Autodesk Inventor part; units mm, degrees
ref_plane "YZ Plane" through (0, 0, 0) normal (1, 0, 0) x (0, 1, 0)
ref_plane "XZ Plane" through (0, 0, 0) normal (0, 1, 0) x (-1, 0, 0)
ref_plane "XY Plane" through (0, 0, 0) normal (0, 0, 1) x (1, 0, 0)
sketch "Sketch1" plane through (0, 0, 0) normal (0, 0, 1) x (1, 0, 0)
  line L0 (0, 4.0415) -> (3.5, 2.0207)
  line L1 (3.5, 2.0207) -> (3.5, -2.0207)
  line L2 (3.5, -2.0207) -> (0, -4.0415)
  line L3 (0, -4.0415) -> (-3.5, -2.0207)
  line L4 (-3.5, -2.0207) -> (-3.5, 2.0207)
  line L5 (-3.5, 2.0207) -> (0, 4.0415)
  point P0 (0, 0)
  point P1 (0, 0)
  dimension "d0" = 7
extrude "Extrusion1" add sketch "Sketch1" along normal blind 2.9
sketch "Sketch2" plane through (0, 0, 2.9) normal (0, 0, 1) x (1, 0, 0)
  circle A0 centre (0, 0) radius 2
  dimension "d3" = 4
extrude "Extrusion2" cut sketch "Sketch2" against normal blind 5
sketch "Sketch3" plane through (0, 0, 2.9) normal (0, 0, 1) x (1, 0, 0)
  circle A0 centre (0, 0) radius 3.5
  circle A1 centre (0, 0) radius 2
extrude "Extrusion3" add sketch "Sketch3" along normal blind 2.1
chamfer "Chamfer1" distance 0.2 angle 45 1 edges at (-2, 0, 0)
thread "Thread1"
chamfer "Chamfer2" distance 0.3 angle 45 1 edges at (-2, 0, 5)
properties part number "P88044_Nylor_Nut_M4"
The listing builds one solid part. Answer for the finished solid, in the listing's coordinates (mm). A direction names the side the tool comes from. Coordinates: 2 decimals unless noted, no trailing zeros. Write each loop counter-clockwise with the first axis right and the second up, starting at its lowest first coordinate (ties: lowest second). Pieces come first, ordered by that corner, then holes. Notation, with made-up numbers: (-2, 59) - (19, 59) arc R28 ccw to (19, 98) - close; hole circle Ø7 at (25, 25). An arc over 180 degrees is marked (long way). Return JSON: item names as keys, results as strings. Group by question number.
1. A cutting plane is placed at A-A, the plane z = 1.45. Determine the outline of the cut face in (x, y), plus the area to 3 significant figures.
2. Which of the six approach directions +Z, -Z, +X, -X, +Y, -Y give full straight-line access (tool end or side, diameter ignored) to faces 1 (the flat face through (-3.15, -1.85, 2.9)), 2 (the flat face through (3.2, -1.8, 2.9)), 3 (the cylindrical face through (3.233, 1.341, 3.935))?
3. A cutting plane is placed at D-D, the plane z = 3.1. Determine the outline of the cut face in (x, y), plus the area to 3 significant figures.
4. A cutting plane is placed at B-B, the plane y = 3.25. Determine the outline of the cut face in (x, z).
5. Straight lines are drawn through the part: L1, parallel to Y at x = 0, z = 3.45; L2, parallel to X at y = -0.5, z = 1.7; L3, parallel to Y at x = -0.75, z = 2.3. For each, find the intervals that lie inside material, in ascending order.
6. Given pin 1 (1.5 mm diameter, centred on x = 1, y = 0.5, fed in from +Z); pin 2 (1.1 mm diameter, centred on x = 0.5, y = 3.5, fed in from +Z); pin 3 (1 mm diameter, centred on x = 1.5, z = 4, fed in from +Y), each flat-ended and moving along its own axis, determine where each tip first touches the part or whether it passes through.
7. Determine the mould class of faces 4 (the cylindrical face through (0, 2, 2)), 5 (the flat face through (-1.726, -3.045, 1.43)), 6 (the flat face through (-3.15, 1.86, 2.9)) for opening direction Y: released by +Y, released by -Y, zero draft, split by the parting line, or undercut.
8. A cutting plane is placed at C-C, the plane x = -2.5. Determine the outline of the cut face in (y, z), plus the area to 3 significant figures.
Ans:
{
 "1": {"outline": "(-3.5, -2.02) - (0, -4.04) - (3.5, -2.02) - (3.5, 2.02) - (0, 4.04) - (-3.5, 2.02) - close; hole circle Ø4 at (0, 0)", "area": "29.9 mm²"},
 "2": {"face 1": "+Z, -X, -Y", "face 2": "+Z, +X, -Y", "face 3": "+Z"},
 "3": {"outline": "circle Ø7 at (0, 0); hole circle Ø4 at (0, 0)", "area": "25.9 mm²"},
 "4": {"outline": "(-1.37, 0) - (1.37, 0) - (1.37, 2.9) - (1.3, 2.9) - (1.3, 5) - (-1.3, 5) - (-1.3, 2.9) - (-1.37, 2.9) - close"},
 "5": {"L1": "-3.5 to -2, 2 to 3.5", "L2": "-3.5 to -1.94, 1.94 to 3.5", "L3": "-3.61 to -1.85, 1.85 to 3.61"},
 "6": {"pin 1": "through", "pin 2": "z = 5", "pin 3": "y = 3.35"},
 "7": {"face 4": "undercut", "face 5": "released by -Y", "face 6": "zero draft"},
 "8": {"outline": "(-2.6, 0) - (2.6, 0) - (2.6, 2.9) - (2.45, 2.9) - (2.45, 5) - (-2.45, 5) - (-2.45, 2.9) - (-2.6, 2.9) - close", "area": "25.4 mm²"}
}
